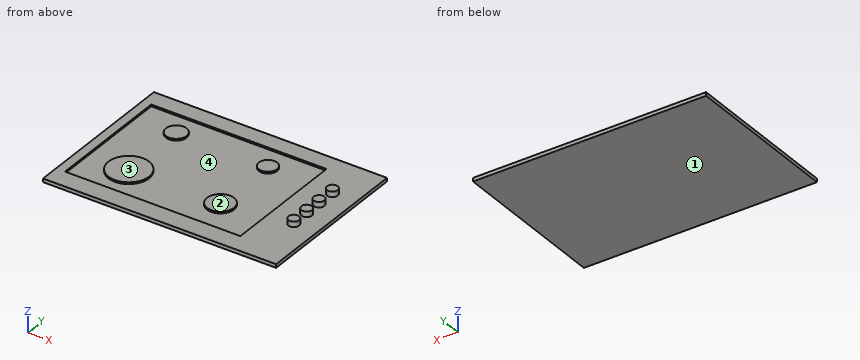
```python
from build123d import *

# Parameters (mm, degrees)
F0_W     = 650
F0_H     = 450
F0_R     = 14.865454
F0_W_2   = 488.997654
F0_H_2   = 349.666808
F1_DEPTH = 10
F0_R_2   = 56.832951
F0_R_3   = 37.769343
F0_R_4   = 28.854156
F0_R_5   = 25.491264
F2_DEPTH = 5
F3_DEPTH = 10
F4_DEPTH = 25


with BuildPart() as f1:
    # F0 (on Top) → F1 (new body)
    with BuildSketch(Plane.XY):
        with Locations((36.786486, -131.776476)):
            Rectangle(F0_W, F0_H)
        with Locations((296.833038, -190.268785)):
            Circle(F0_R, mode=Mode.SUBTRACT)
        with Locations((296.833038, -138.121739)):
            Circle(F0_R, mode=Mode.SUBTRACT)
        with Locations((-18.782042, -128.970219)):
            Rectangle(F0_W_2, F0_H_2, mode=Mode.SUBTRACT)
        with Locations((296.833038, -88.088758)):
            Circle(F0_R, mode=Mode.SUBTRACT)
        with Locations((296.833038, -33.827644)):
            Circle(F0_R, mode=Mode.SUBTRACT)
    extrude(amount=F1_DEPTH)

    # F0 (on Top) → F2 (join)
    with BuildSketch(Plane.XY):
        with Locations((-18.782042, -128.970219)):
            Rectangle(F0_W_2, F0_H_2)
        with Locations((-148.592174, -211.847812)):
            Circle(F0_R_2, mode=Mode.SUBTRACT)
        with Locations((107.138157, -211.847812)):
            Circle(F0_R_3, mode=Mode.SUBTRACT)
        with Locations((-148.592174, -19.205136)):
            Circle(F0_R_4, mode=Mode.SUBTRACT)
        with Locations((107.138157, -19.205136)):
            Circle(F0_R_5, mode=Mode.SUBTRACT)
    extrude(amount=F2_DEPTH)

    # F0 (on Top) → F3 (join)
    with BuildSketch(Plane.XY):
        with Locations((-148.592174, -19.205136)):
            Circle(F0_R_4)
        with Locations((107.138157, -19.205136)):
            Circle(F0_R_5)
        with Locations((107.138157, -211.847812)):
            Circle(F0_R_3)
        with Locations((-148.592174, -211.847812)):
            Circle(F0_R_2)
    extrude(amount=F3_DEPTH)

    # F0 (on Top) → F4 (join)
    with BuildSketch(Plane.XY):
        with Locations((296.833038, -33.827644)):
            Circle(F0_R)
        with Locations((296.833038, -88.088758)):
            Circle(F0_R)
        with Locations((296.833038, -138.121739)):
            Circle(F0_R)
        with Locations((296.833038, -190.268785)):
            Circle(F0_R)
    extrude(amount=F4_DEPTH)


solid = f1.part
```
Could you check a few things on this model? Use its own coordinates, in mm. Face numbers are marked on the shaded views. A direction names the side the tool comes from. Round coordinates to 2 decimals unless told otherwise and drop trailing zeros. Order: outer loops, then holes, each group sorted by start corner. A loop starts at its lowest first (then second) coordinate and runs counter-clockwise, first axis right, second up. Notation, with made-up numbers: (32, -10) -> (71, -10) arc R22 cw to (71, 7) -> close; hole circle Ø2 at (37, 12). An arc over 180 degrees is marked (long way). One line per question, with ' | ' between items.
Q1. I'm going to push flat-ended pins straight in: pin 1 (1.5 mm diameter, centred on x = 226, y = -231.5, fed in from -Z); pin 2 (17.5 mm diameter, centred on x = -138.5, y = -9, fed in from +Z); pin 3 (10 mm diameter, centred on x = 23.5, y = -56.5, fed in from +Z); pin 4 (8 mm diameter, centred on y = -152, z = 17.5, fed in from +X). Where does each tip first touch, or does it pass through?
Computed values:
pin 1: z = 0 | pin 2: z = 10 | pin 3: z = 5 | pin 4: x = 307.94
Q2. If we section it at D-D on x = 244: Write out the boundary of the cut face in (y, z).
Computed values:
outline: (-356.78, 0) -> (93.22, 0) -> (93.22, 10) -> (-356.78, 10) -> close
Q3. Which directions (+Z, -Z, +X, -X, +Y, -Y) give clear straight access to the entire face, cutting with the end or side of a thin tool? Please do the marked faces 1 and 2.
Computed values:
face 1: -Z, +X, -X, +Y, -Y | face 2: +Z, -X, +Y, -Y
Q4. If I drill on line 1 (X direction, y = -298, z = 6); line 2 (Y direction, x = 294.5, z = 23.75); line 3 (Z direction, x = -111, y = 42.5), over which ranges is the centre line in solid material (lowest first)? Write a range as from..to.
Computed values:
line 1: -288.21..-263.28, 225.72..361.79 | line 2: -204.95..-175.59, -152.8..-123.44, -102.77..-73.41, -48.51..-19.15 | line 3: 0..5
Q5. If we section it at C-C on z = 17.5: Write out the boundary of the cut face in (x, y).
Computed values:
outline: circle Ø29.73 at (296.83, -190.27); circle Ø29.73 at (296.83, -138.12); circle Ø29.73 at (296.83, -88.09); circle Ø29.73 at (296.83, -33.83)
Q6. If we section it at B-B on x = -38.5: Write out the boundary of the cut face in (y, z), plus the area to 3 significant figures.
Computed values:
outline: (-356.78, 0) -> (93.22, 0) -> (93.22, 10) -> (45.86, 10) -> (45.86, 5) -> (-303.8, 5) -> (-303.8, 10) -> (-356.78, 10) -> close | area: 2,750 mm²
Q7. We'd pull the mould along Y, two halves only. Please class the marked faces 3 and 4: released by +Y, released by -Y, zero draft, split by the parting line, or undercut.
Computed values:
face 3: zero draft | face 4: undercut
Q8. If we section it at A-A on y = -66: Write out the boundary of the cut face in (x, z).
Computed values:
outline: (-288.21, 0) -> (361.79, 0) -> (361.79, 10) -> (225.72, 10) -> (225.72, 5) -> (-263.28, 5) -> (-263.28, 10) -> (-288.21, 10) -> close
